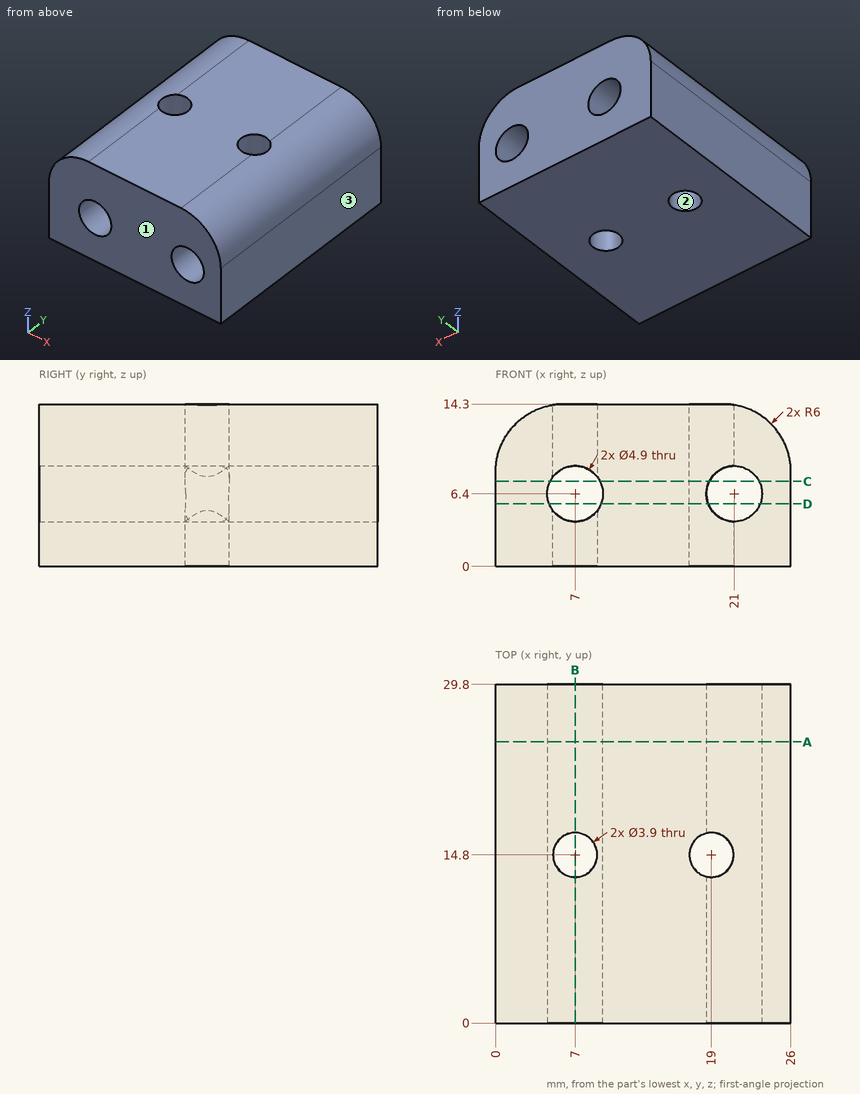
Check sheet for the drawn part. Datum: minimum x, y, z corner. Units: mm. Coordinates: 2 decimals unless noted, no trailing zeros. Write each loop counter-clockwise with the first axis right and the second up, starting at its lowest first coordinate (ties: lowest second). Pieces come first, ordered by that corner, then holes. Notation, with made-up numbers: M 36,-17 L 88,-17 A24 ccw 88,8 Z; hole C 44.25,-29.75 d6. An arc over 180 degrees is marked long. Use a Markdown table: item, result.
Q1. Draft check along Y on the marked faces 1, 2 and 3. Enter one of: +Y half, -Y half, draft (parallel to the pull), parting line (faces both ways), or undercut.
Reply:
| item | result |
|---|---|
| face 1 | -Y half |
| face 2 | undercut |
| face 3 | draft |
Q2. Go/stop test with flat-tipped pins: P1, Ø2, axis at y = 4.5, z = 12.5, coming from the -X side; P2, Ø5.5, axis at x = 21, z = 6.4, coming from the -Y side; P3, Ø2, axis at y = 4.5, z = 12, coming from the -X side. Record where each tip stops, or that it passes through.
Reply:
| item | result |
|---|---|
| P1 | stops at x = 0.92 |
| P2 | stops at y = 0 |
| P3 | stops at x = 0.64 |
Q3. Sectioned sample at A-A, the plane y = 24.75. Record the boundary of the cut face in (x, z).
Reply:
| item | result |
|---|---|
| outline | M 0,0 L 26,0 L 26,8.3 A6 ccw 20,14.3 L 6,14.3 A6 ccw 0,8.3 Z; hole C 7,6.4 d4.9; hole C 21,6.4 d4.9 |
Q4. Sectioned sample at B-B, the plane x = 7. Record the boundary of the cut face in (y, z).
Reply:
| item | result |
|---|---|
| outline | M 0,0 L 12.85,0 L 12.85,3.95 L 0,3.95 Z; M 0,8.85 L 12.85,8.85 L 12.85,14.3 L 0,14.3 Z; M 16.75,0 L 29.8,0 L 29.8,3.95 L 16.75,3.95 Z; M 16.75,8.85 L 29.8,8.85 L 29.8,14.3 L 16.75,14.3 Z |
Q5. Sectioned sample at D-D, the plane z = 5.5. Record the boundary of the cut face in (x, y).
Reply:
| item | result |
|---|---|
| outline | M 0,0 L 4.72,0 L 4.72,29.8 L 0,29.8 Z; M 9.28,0 L 18.72,0 L 18.72,12.87 A1.95 cw 18.72,16.73 L 18.72,29.8 L 9.28,29.8 Z; M 23.28,0 L 26,0 L 26,29.8 L 23.28,29.8 Z |
Q6. Sectioned sample at C-C, the plane z = 7.5. Record the boundary of the cut face in (x, y).
Reply:
| item | result |
|---|---|
| outline | M 0,0 L 4.81,0 L 4.81,29.8 L 0,29.8 Z; M 9.19,0 L 18.81,0 L 18.81,12.86 A1.95 cw 18.81,16.74 L 18.81,29.8 L 9.19,29.8 Z; M 23.19,0 L 26,0 L 26,29.8 L 23.19,29.8 Z |
Q7. Thickness scan on line 1 (Y direction, x = 19, z = 8.75); line 2 (X direction, y = 14.8, z = 7); line 3 (X direction, y = 1.75, z = 5.5). Record the ranges inside material, lowest first.
Reply:
| item | result |
|---|---|
| line 1 | y = 0 to 12.85, 16.75 to 29.8 |
| line 2 | x = 0 to 4.62, 9.38 to 17.05, 23.38 to 26 |
| line 3 | x = 0 to 4.72, 9.28 to 18.72, 23.28 to 26 |
